Input: part model. Units: mm. Frame: model coordinates. Face numbers are marked on the shaded views. Give positions to 0.01 mm unless a question says otherwise; leave off trailing zeros. Loops run counter-clockwise (first coordinate to the right, second up) from the corner with the lowest first, then second, coordinate; pieces in that order, holes last. Notation, with made-up numbers: (20, 8.25) - (52, 8.25) arc R19 ccw to (52, 12.25) - close; hole circle Ø10 at (5.5, 74.25). An arc over 180 degrees is marked (long way). Answer as a JSON object with one key per item and string values. Group by question number.
(1) Section query D-D (x = 0.75). Return loops of the section in (y, z), plus the area to 3 significant figures.
(2) Material intervals for L1, parallel to Y at x = 1.5, z = -0.3; L2, parallel to X at y = 0.3, z = -0.15; L3, parallel to Y at x = -1.25, z = -0.45, sorted ascending.
(3) Section query C-C (z = -0.3). Return loops of the section in (x, y), plus the area to 3 significant figures.
(4) Section query B-B (x = -1.5). Return loops of the section in (y, z), plus the area to 3 significant figures.
(5) Mould query, pull axis X, two halves, no side actions, for the marked faces 1, 2, 3 and 4. Classes: +X half, -X half, draft (parallel to the pull), parting line (faces both ways), or undercut.
(6) Section query A-A (y = 0.5). Return loops of the section in (x, z), plus the area to 3 significant figures.
```python
from build123d import *

# Parameters (mm, degrees)
BOSS_EXTRUDE1_DEPTH            = 0.5
SKETCH2_R                      = 2.3
CUT_EXTRUDE1_DEPTH             = 1.5
CUT_EXTRUDE2_DEPTH             = 1.5
F_0_8_0_8_DIAMETER_HOLE1_D     = 0.8
F_0_8_0_8_DIAMETER_HOLE1_DEPTH = 0.5


with BuildPart() as part:
    # Sketch1 → Boss-Extrude1 (new body)
    with BuildSketch(Plane.XY):
        with BuildLine():
            Line((-2.5, 2.890366769), (-2.5, 1.833030278))
            ThreePointArc((-2.5, 1.833030278), (0, -3.1), (2.5, 1.833030278))
            Line((2.5, 1.833030278), (2.5, 2.890366769))
            ThreePointArc((2.5, 2.890366769), (0, 3.9), (-2.5, 2.890366769))
        make_face()
    extrude(amount=-BOSS_EXTRUDE1_DEPTH)

    # Sketch2 → Cut-Extrude1 (cut, through all)
    with BuildSketch(Plane.XY):
        with Locations((0, 0.3)):
            Circle(SKETCH2_R)
    extrude(amount=-CUT_EXTRUDE1_DEPTH, mode=Mode.SUBTRACT)

    # Sketch3 → Cut-Extrude2 (cut, through all)
    with BuildSketch(Plane.XY):
        with BuildLine():
            Line((-0.42, 3.87541606), (-0.42, 2.561327044))
            ThreePointArc((-0.42, 2.561327044), (0, 2.6), (0.42, 2.561327044))
            Line((0.42, 2.561327044), (0.42, 3.87541606))
            ThreePointArc((0.42, 3.87541606), (0, 3.9), (-0.42, 3.87541606))
        make_face()
    extrude(amount=-CUT_EXTRUDE2_DEPTH, mode=Mode.SUBTRACT)

    # Ø0.8 (0.8) Diameter Hole1
    with Locations(Plane.XY):
        with Locations((-1.5, 2.898076211), (1.5, 2.898076211)):
            Hole(F_0_8_0_8_DIAMETER_HOLE1_D / 2, depth=F_0_8_0_8_DIAMETER_HOLE1_DEPTH)


solid = part.part
```
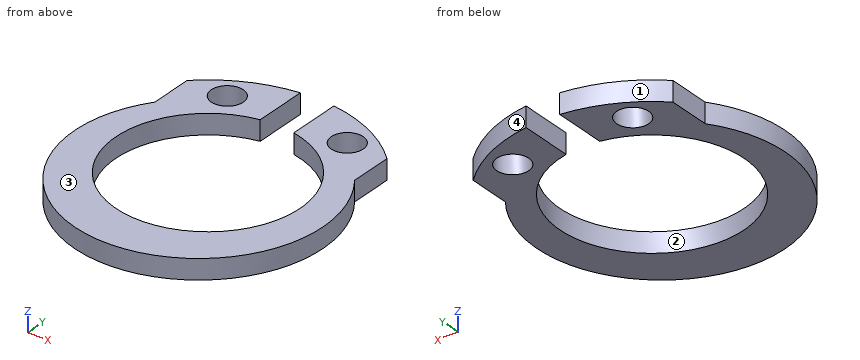
Recorded:
{
 "1": {"outline": "(-3.01, -0.5) - (-1.87, -0.5) - (-1.87, 0) - (-3.01, 0) - close; (2.47, -0.5) - (3.82, -0.5) - (3.82, 0) - (2.47, 0) - close", "area": "1.24 mm^2"},
 "2": {"L1": "y = -2.71 to -1.44, 2.04 to 2.5, 3.3 to 3.57", "L2": "x = -3.09 to -2.3, 2.3 to 3.09", "L3": "y = -2.84 to -1.63, 2.23 to 2.59, 3.21 to 3.68"},
 "3": {"outline": "(-2.5, 1.83) arc R3.1 ccw (long way) to (2.5, 1.83) - (2.5, 2.89) arc R3.6 ccw to (0.42, 3.88) - (0.42, 2.56) arc R2.3 cw (long way) to (-0.42, 2.56) - (-0.42, 3.88) arc R3.6 ccw to (-2.5, 2.89) - close; hole circle Ø0.8 at (-1.5, 2.9); hole circle Ø0.8 at (1.5, 2.9)", "area": "15.8 mm^2"},
 "4": {"outline": "(-2.71, -0.5) - (-1.44, -0.5) - (-1.44, 0) - (-2.71, 0) - close; (2.04, -0.5) - (2.5, -0.5) - (2.5, 0) - (2.04, 0) - close; (3.3, -0.5) - (3.57, -0.5) - (3.57, 0) - (3.3, 0) - close", "area": "0.999 mm^2"},
 "5": {"face 1": "-X half", "face 2": "undercut", "face 3": "draft", "face 4": "+X half"},
 "6": {"outline": "(-3.06, -0.5) - (-2.29, -0.5) - (-2.29, 0) - (-3.06, 0) - close; (2.29, -0.5) - (3.06, -0.5) - (3.06, 0) - (2.29, 0) - close", "area": "0.768 mm^2"}
}
